Work out the finished part from the listing and answer in its coordinate system (mm). Face numbers are marked on the shaded views. A direction names the side the tool comes from. Give positions to 0.01 mm unless a question says otherwise; leave off trailing zeros. Write each loop counter-clockwise with the first axis right and the second up, starting at its lowest first coordinate (ties: lowest second). Pieces come first, ordered by that corner, then holes. Notation, with made-up numbers: (-21.5, 62.5) - (20.5, 62.5) arc R16 cw to (20.5, 76.5) - close; hole circle Ø2 at (48, -3). An arc over 180 degrees is marked (long way). Write each question's results on one line, items separated by ' | '. Start each with the question number.
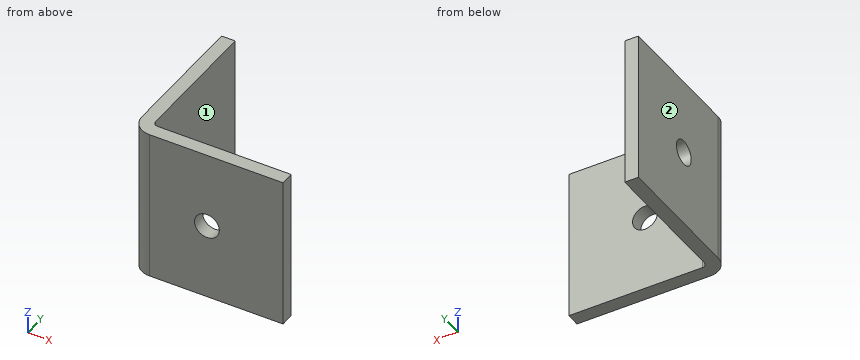
from build123d import *

# Parameters (mm, degrees)
SKETCH1_W                  = 25.4
SKETCH1_H                  = 1498.6
BOSS_EXTRUDE1_DEPTH        = 25.4
SKETCH2_W                  = 23.114
SKETCH2_H                  = 23.114
CUT_EXTRUDE1_DEPTH         = 1499.6
M3_5_CLEARANCE_HOLE1_D     = 4.1402
M3_5_CLEARANCE_HOLE1_DEPTH = 25.4
M3_5_CLEARANCE_HOLE2_D     = 4.1402
M3_5_CLEARANCE_HOLE2_DEPTH = 25.4
CHAMFER1_SIZE              = 2.159
FILLET1_R                  = 0.8128
FILLET2_R                  = 3.0988
SKETCH8_W                  = 95.882963774
SKETCH8_H                  = 79.338329604
CUT_EXTRUDE3_DEPTH         = 1371.6
SKETCH9_W                  = 56.924523055
SKETCH9_H                  = 51.282783217
CUT_EXTRUDE4_DEPTH         = 76.2
SKETCH10_W                 = 57.247248429
SKETCH10_H                 = 53.712272172
CUT_EXTRUDE5_DEPTH         = 25.4


with BuildPart() as part:
    # Sketch1 → Boss-Extrude1 (new body)
    with BuildSketch(Plane(origin=(0, 0, 0), x_dir=(0, -1, 0), z_dir=(-1, 0, 0))):
        with Locations((-12.7, 0)):
            Rectangle(SKETCH1_W, SKETCH1_H)
    extrude(amount=-BOSS_EXTRUDE1_DEPTH)

    # Sketch2 → Cut-Extrude1 (cut, through all)
    with BuildSketch(Plane(origin=(0, 0, -749.3), x_dir=(-1, 0, 0), z_dir=(0, 0, -1))):
        with Locations((-13.843, 13.843)):
            Rectangle(SKETCH2_W, SKETCH2_H)
    extrude(amount=-CUT_EXTRUDE1_DEPTH, mode=Mode.SUBTRACT)

    # M3.5 Clearance Hole1
    with Locations(Plane(origin=(0, 0, 0), x_dir=(-1, 0, 0), z_dir=(0, -1, 0))):
        with Locations((-12.7, 736.6), (-12.7, 711.2), (-12.7, 685.8), (-12.7, 660.4), (-12.7, 635), (-12.7, 609.6), (-12.7, 584.2), (-12.7, 558.8), (-12.7, 533.4), (-12.7, 508), (-12.7, 482.6), (-12.7, 457.2), (-12.7, 431.8), (-12.7, 406.4), (-12.7, 381), (-12.7, 355.6), (-12.7, 330.2), (-12.7, 304.8), (-12.7, 279.4), (-12.7, 254), (-12.7, 228.6), (-12.7, 203.2), (-12.7, 177.8), (-12.7, 152.4), (-12.7, 127), (-12.7, 101.6), (-12.7, 76.2), (-12.7, 50.8), (-12.7, 25.4), (-12.7, 0), (-12.7, -25.4), (-12.7, -50.8), (-12.7, -76.2), (-12.7, -101.6), (-12.7, -127), (-12.7, -152.4), (-12.7, -177.8), (-12.7, -203.2), (-12.7, -228.6), (-12.7, -254), (-12.7, -279.4), (-12.7, -304.8), (-12.7, -330.2), (-12.7, -355.6), (-12.7, -381), (-12.7, -406.4), (-12.7, -431.8), (-12.7, -457.2), (-12.7, -482.6), (-12.7, -508), (-12.7, -533.4), (-12.7, -558.8), (-12.7, -584.2), (-12.7, -609.6), (-12.7, -635), (-12.7, -660.4), (-12.7, -685.8), (-12.7, -711.2), (-12.7, -736.6)):
            Hole(M3_5_CLEARANCE_HOLE1_D / 2, depth=M3_5_CLEARANCE_HOLE1_DEPTH)

    # M3.5 Clearance Hole2
    with Locations(Plane.ZY):
        with Locations((711.2, 12.7), (736.6, 12.7), (685.8, 12.7), (660.4, 12.7), (635, 12.7), (609.6, 12.7), (584.2, 12.7), (558.8, 12.7), (533.4, 12.7), (508, 12.7), (482.6, 12.7), (457.2, 12.7), (431.8, 12.7), (406.4, 12.7), (381, 12.7), (355.6, 12.7), (330.2, 12.7), (304.8, 12.7), (279.4, 12.7), (254, 12.7), (228.6, 12.7), (203.2, 12.7), (177.8, 12.7), (152.4, 12.7), (127, 12.7), (101.6, 12.7), (76.2, 12.7), (50.8, 12.7), (25.4, 12.7), (0, 12.7), (-25.4, 12.7), (-50.8, 12.7), (-76.2, 12.7), (-101.6, 12.7), (-127, 12.7), (-152.4, 12.7), (-177.8, 12.7), (-203.2, 12.7), (-228.6, 12.7), (-254, 12.7), (-279.4, 12.7), (-304.8, 12.7), (-330.2, 12.7), (-355.6, 12.7), (-381, 12.7), (-406.4, 12.7), (-431.8, 12.7), (-457.2, 12.7), (-482.6, 12.7), (-508, 12.7), (-533.4, 12.7), (-558.8, 12.7), (-584.2, 12.7), (-609.6, 12.7), (-635, 12.7), (-660.4, 12.7), (-685.8, 12.7), (-711.2, 12.7), (-736.6, 12.7)):
            Hole(M3_5_CLEARANCE_HOLE2_D / 2, depth=M3_5_CLEARANCE_HOLE2_DEPTH)

    # Chamfer1
    chamfer1_edges = [part.edges().sort_by_distance(p)[0] for p in [
        (25.4, 1.143, -749.3),
        (1.143, 25.4, 749.3),
        (1.143, 25.4, -749.3),
        (25.4, 1.143, 749.3),
    ]]
    chamfer(chamfer1_edges, length=CHAMFER1_SIZE)

    # Fillet1
    fillet1_edges = [part.edges().sort_by_distance(p)[0] for p in [
        (2.286, 2.286, 0),
    ]]
    fillet(fillet1_edges, radius=FILLET1_R)

    # Fillet2
    fillet2_edges = [part.edges().sort_by_distance(p)[0] for p in [
        (0, 0, 0),
    ]]
    fillet(fillet2_edges, radius=FILLET2_R)

    # Sketch8 → Cut-Extrude3 (cut)
    with BuildSketch(Plane.XY.offset(749.3)):
        with Locations((2.286, 3.0988)):
            Rectangle(SKETCH8_W, SKETCH8_H)
    extrude(amount=-CUT_EXTRUDE3_DEPTH, mode=Mode.SUBTRACT)

    # Sketch9 → Cut-Extrude4 (cut)
    with BuildSketch(Plane(origin=(0, 0, -749.3), x_dir=(-1, 0, 0), z_dir=(0, 0, -1))):
        with Locations((-2.180776643, 1.30746368)):
            Rectangle(SKETCH9_W, SKETCH9_H)
    extrude(amount=-CUT_EXTRUDE4_DEPTH, mode=Mode.SUBTRACT)

    # Sketch10 → Cut-Extrude5 (cut)
    with BuildSketch(Plane.XY.offset(-622.3)):
        with Locations((2.141729058, 1.213934322)):
            Rectangle(SKETCH10_W, SKETCH10_H)
    extrude(amount=-CUT_EXTRUDE5_DEPTH, mode=Mode.SUBTRACT)


solid = part.part
Q1. A tool of negligible diameter and unlimited length cuts with its end or side. For the marked faces 1 and 2, from which of +Z, -Z, +X, -X, +Y, -Y can it reach the whole face along a straight path? Write none if from no direction.
Q2. Given pin 1 (2 mm diameter, centred on y = 16.5, z = -663.5, fed in from +X); pin 2 (3.5 mm diameter, centred on y = 12.7, z = -660.4, fed in from +X), each flat-ended and moving along its own axis, determine where each tip first touches the part or whether it passes through.
Q3. A cutting plane is placed at A-A, the plane y = 12.7. Write down the section's boundary in (x, z).
Q4. A cutting plane is placed at C-C, the plane z = -660.4. Write down the section's boundary in (x, y), and give its area (3 significant figures).
Q5. A cutting plane is placed at D-D, the plane z = -651.25. Write down the section's boundary in (x, y), and give its area (3 significant figures).
Q6. Consider L1, parallel to Z at x = 12.7, y = 1.6; L2, parallel to Y at x = 12.75, z = -657.25. Determine where each line is inside the solid, lowest interval first.
Result:
1) face 1: +Z, -Z, +X, +Y | face 2: +Z, -Z, -X, +Y, -Y
2) pin 1: stops at x = 2.29 | pin 2: passes through
3) outline: (0, -673.1) - (2.29, -673.1) - (2.29, -662.47) - (0, -662.47) - close; (0, -658.33) - (2.29, -658.33) - (2.29, -647.7) - (0, -647.7) - close
4) outline: (0, 3.1) arc R3.1 ccw to (3.1, 0) - (10.63, 0) - (10.63, 2.29) - (3.1, 2.29) arc R0.81 cw to (2.29, 3.1) - (2.29, 10.63) - (0, 10.63) - close; (0, 14.77) - (2.29, 14.77) - (2.29, 25.4) - (0, 25.4) - close; (14.77, 0) - (25.4, 0) - (25.4, 2.29) - (14.77, 2.29) - close | area: 90.1 mm2
5) outline: (0, 3.1) arc R3.1 ccw to (3.1, 0) - (25.4, 0) - (25.4, 2.29) - (3.1, 2.29) arc R0.81 cw to (2.29, 3.1) - (2.29, 25.4) - (0, 25.4) - close | area: 109 mm2
6) L1: z = -673.1 to -662.47, -658.33 to -647.7 | L2: y = 0 to 2.29
